Could you check a few things on this model? Use its own coordinates, in mm. Round coordinates to 2 decimals unless told otherwise and drop trailing zeros. Loops run counter-clockwise (first coordinate to the right, second up) from the corner with the lowest first, then second, coordinate; pieces in that order, holes last. Notation, with made-up numbers: (35.25, 49.25) -> (46.25, 49.25) arc R21 ccw to (46.25, 57.25) -> close; hole circle Ø6 at (14.5, 31.5). An arc over 180 degrees is marked (long way). One line per item, written item: value.
Autodesk Inventor part; units mm, degrees
ref_plane "YZ Plane" through (0, 0, 0) normal (1, 0, 0) x (0, 1, 0)
ref_plane "XZ Plane" through (0, 0, 0) normal (0, 1, 0) x (-1, 0, 0)
ref_plane "XY Plane" through (0, 0, 0) normal (0, 0, 1) x (1, 0, 0)
sketch "草圖1" plane through (0, 0, 0) normal (0, 1, 0) x (-1, 0, 0)
  arc A0 (0, -25) -> (0, 25) centre (0, 0) ccw
  line L0 (0, -25) -> (-300, -25)
  line L1 (-300, -25) -> (-300, 25) construction
  line L2 (-300, 25) -> (0, 25)
  line L3 (0, 25) -> (0, -25) construction
  arc A1 (-300, 25) -> (-300, -25) centre (-300, 0) ccw
  dimension "diameter" = 50
  dimension "center_length" = 300
extrude "thickness" add sketch "草圖1" along normal blind 10
sketch "草圖2" plane through (0, 10, 0) normal (0, 1, 0) x (1, 0, 0)
  circle A0 centre (0, 0) radius 12.5
  arc A1 (0, 25) -> (0, -25) centre (0, 0) ccw construction
  line L0 (0, -25) -> (300, -25) construction
  arc A2 (300, -25) -> (300, 25) centre (300, 0) ccw construction
  line L1 (300, 25) -> (0, 25) construction
  circle A3 centre (300, 0) radius 12.5
  dimension "hole" = 25
extrude "擠出2" cut sketch "草圖2" against normal up to surface (10 mm away)
properties part number "test"
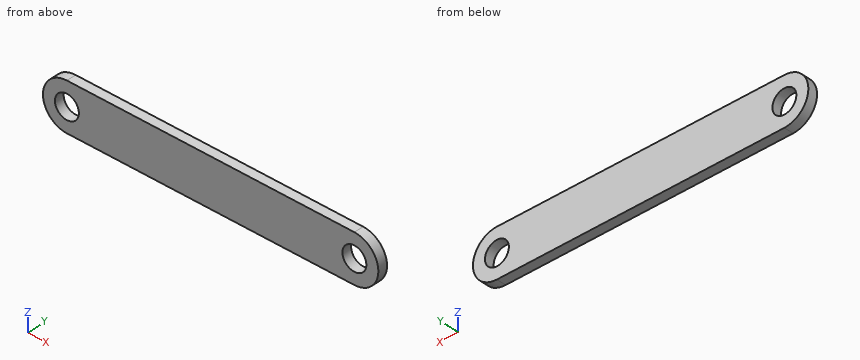
(1) Imagine slicing it at D-D on z = 9. Write out the boundary of the cut face in (x, y), then the cut area to 3 significant figures.
Results below:
outline: (-23.32, 0) -> (-8.67, 0) -> (-8.67, 10) -> (-23.32, 10) -> close; (8.67, 0) -> (291.33, 0) -> (291.33, 10) -> (8.67, 10) -> close; (308.67, 0) -> (323.32, 0) -> (323.32, 10) -> (308.67, 10) -> close
area: 3,120 mm²
(2) For pin 1 Ø1 at (y, z) = (6, -16.5) entering from -X; pin 2 Ø3 at (x, z) = (96.5, 9) entering from -Y; pin 3 Ø22.5 at (x, z) = (300, 0) entering from +Y, each with a flat end and sliding along its axis, tell me the tip position at first contact or that it passes through.
Results below:
pin 1: stops at x = -19.21
pin 2: stops at y = 0
pin 3: passes through
(3) Imagine slicing it at B-B on x = 294.5. Write out the boundary of the cut face in (y, z), then the cut area to 4 significant figures.
Results below:
outline: (0, -25) -> (10, -25) -> (10, -11.22) -> (0, -11.22) -> close; (0, 11.22) -> (10, 11.22) -> (10, 25) -> (0, 25) -> close
area: 275.5 mm²
(4) Please list where these lines run through material, in increasing order: L1, parallel to X at y = 4.25, z = 0; L2, parallel to Z at x = 0, y = 6; L3, parallel to X at y = 7, z = 1.5.
Results below:
L1: x = -25 to -12.5, 12.5 to 287.5, 312.5 to 325
L2: z = -25 to -12.5, 12.5 to 25
L3: x = -24.95 to -12.41, 12.41 to 287.59, 312.41 to 324.95
(5) Imagine slicing it at C-C on z = -4. Write out the boundary of the cut face in (x, y), then the cut area to 3 significant figures.
Results below:
outline: (-24.68, 0) -> (-11.84, 0) -> (-11.84, 10) -> (-24.68, 10) -> close; (11.84, 0) -> (288.16, 0) -> (288.16, 10) -> (11.84, 10) -> close; (311.84, 0) -> (324.68, 0) -> (324.68, 10) -> (311.84, 10) -> close
area: 3,020 mm²
(6) Imagine slicing it at A-A on y = 7.75. Write out the boundary of the cut face in (x, z).
Results below:
outline: (0, -25) -> (300, -25) arc R25 ccw to (300, 25) -> (0, 25) arc R25 ccw to start; hole circle Ø25 at (0, 0); hole circle Ø25 at (300, 0)
